The model under review builds one solid part; all positions refer to its coordinate system, in mm. A direction names the side the tool comes from. Round coordinates to 2 decimals unless told otherwise and drop trailing zeros. Write each loop counter-clockwise with the first axis right and the second up, starting at its lowest first coordinate (ties: lowest second). Pieces come first, ordered by that corner, then holes. Notation, with made-up numbers: (-18.5, 59) - (25.5, 59) arc R14 ccw to (25.5, 75) - close; hole circle Ø3 at (71.5, 46). An arc over 180 degrees is marked (long way). Return JSON: item names as keys, results as strings.
Autodesk Fusion 360 part; units mm, degrees
sketch "Sketch1" plane through (0, 0, 0) normal (0, 1, 0) x (1, 0, 0)
  line L0 (0, 0) -> (40.47, 0)
  line L1 (40.47, 0) -> (40.47, -39.36)
  line L2 (40.47, -39.36) -> (0, -39.36)
  line L3 (0, -39.36) -> (0, 0)
  line L4 (40.47, -9.96) -> (47.35, -9.96)
  line L5 (47.35, -9.96) -> (47.35, -12.36)
  line L6 (47.35, -12.36) -> (40.47, -12.36)
  line L7 (40.47, -29.96) -> (46.47, -29.96)
  line L8 (46.47, -29.96) -> (46.47, -33.96)
  line L9 (46.47, -33.96) -> (40.47, -33.96)
  line L10 (20.235, 0) -> (20.235, -39.36) construction
  line L11 (0, -9.96) -> (-6.88, -9.96)
  line L12 (-6.88, -9.96) -> (-6.88, -12.36)
  line L13 (-6.88, -12.36) -> (0, -12.36)
  dimension "d1" = 40.47
  dimension "d2" = 39.36
  dimension "d3" = 6.88
  dimension "d4" = 2.4
  dimension "d5" = 27
  dimension "d6" = 6
  dimension "d7" = 4
  dimension "d8" = 5.4
extrude "Extrude1" add sketch "Sketch1" along normal blind 19.6
sketch "Sketch2" plane through (0, 0, 0) normal (0, 0, -1) x (-1, 0, 0)
  line L0 (-40.47, 0) -> (0, 0)
  line L1 (0, 0) -> (0, 19.6)
  line L2 (0, 19.6) -> (-40.47, 19.6)
  line L3 (-40.47, 19.6) -> (-40.47, 0)
  circle A0 centre (-30.8, 9.8) radius 2.92
  line L4 (0, 9.8) -> (-40.47, 9.8) construction
  dimension "d11" = 5.84
  dimension "d12" = 9.67
extrude "Extrude2" add sketch "Sketch2" along normal blind 3.81 contours A0
sketch "Sketch3" plane through (0, 0, 9.96) normal (0, 0, -1) x (-1, 0, 0)
  line L0 (-47.35, 0) -> (-40.47, 0)
  line L1 (-40.47, 0) -> (-40.47, 19.6)
  line L2 (-40.47, 19.6) -> (-47.35, 19.6)
  line L3 (-47.35, 19.6) -> (-47.35, 0)
  circle A0 centre (-44.425, 14.58) radius 1.915
  circle A1 centre (-44.425, 5.02) radius 1.915
  line L4 (-40.47, 9.8) -> (-47.35, 9.8) construction
  line L5 (-40.47, 0) -> (-40.47, 19.6)
  line L6 (0, 0) -> (0, 19.6)
  line L7 (0, 0) -> (-40.47, 0)
  line L8 (-40.47, 19.6) -> (0, 19.6)
  line L9 (-20.235, 19.6) -> (-20.235, 0) construction
  dimension "d15" = 3.83
  dimension "d16" = 3.83
  dimension "d17" = 9.56
  dimension "d19" = 2.925
extrude "Extrude3" cut sketch "Sketch3" against normal up to surface (2.4 mm away) contours A0 | A1
ref_plane "WorkPlane1" through (20.235, 9.8, 4.98) normal (-1, 0, 0) x (0, 0, 1)
mirror "Mirror1" about plane through (20.235, 9.8, 4.98) normal (-1, 0, 0) of "Extrude3"
(1) Wall thickness on line 1 (Z direction, x = 35.5, y = 3.5); line 2 (X direction, y = 3.75, z = 28); line 3 (X direction, y = 2.5, z = 33.5): over which ranges is each line inside the solid? List them lowest first.
Filled in:
{"line 1": "z = 0 to 39.36", "line 2": "x = 0 to 40.47", "line 3": "x = 0 to 46.47"}
(2) Add section A-A (y = 5.02). Write out the cut boundary in (x, z).
Filled in:
{"outline": "(-6.88, 9.96) - (-5.87, 9.96) - (-5.87, 12.36) - (-6.88, 12.36) - close; (-2.04, 9.96) - (0, 9.96) - (0, 0) - (40.47, 0) - (40.47, 9.96) - (42.51, 9.96) - (42.51, 12.36) - (40.47, 12.36) - (40.47, 29.96) - (46.47, 29.96) - (46.47, 33.96) - (40.47, 33.96) - (40.47, 39.36) - (0, 39.36) - (0, 12.36) - (-2.04, 12.36) - close; (46.34, 9.96) - (47.35, 9.96) - (47.35, 12.36) - (46.34, 12.36) - close"}
(3) Clearance check with flat-ended pins moving along their axes: pin 1 Ø6 at (y, z) = (13, 25) entering from -X; pin 2 Ø8 at (y, z) = (12, 5.5) entering from +X; pin 3 Ø3.5 at (x, y) = (-3, 10) entering from -Z; pin 4 Ø3 at (x, y) = (-3.955, 14.58) entering from -Z. State where each tip first meets the part, or that it passes through.
Filled in:
{"pin 1": "stops at x = 0", "pin 2": "stops at x = 40.47", "pin 3": "stops at z = 9.96", "pin 4": "passes through"}
(4) Add section C-C (y = 17.75). Write out the cut boundary in (x, z), plus the area to 3 significant figures.
Filled in:
{"outline": "(-6.88, 9.96) - (0, 9.96) - (0, 0) - (40.47, 0) - (40.47, 9.96) - (47.35, 9.96) - (47.35, 12.36) - (40.47, 12.36) - (40.47, 29.96) - (46.47, 29.96) - (46.47, 33.96) - (40.47, 33.96) - (40.47, 39.36) - (0, 39.36) - (0, 12.36) - (-6.88, 12.36) - close", "area": "1,650 mm2"}
(5) Mouldability with a two-part tool opening along Y and no side actions: class faces 5 (the flat face through (20, 19.6, 19)), 6 (the flat face through (20, 0, 19)), 7 (the flat face through (-3, 10, 12.36)), 8 (the cylindrical face through (42.6, 15.16, 11.14)) as released by +Y, released by -Y, zero draft, split by the parting line, or undercut.
Filled in:
{"face 5": "released by +Y", "face 6": "released by -Y", "face 7": "zero draft", "face 8": "undercut"}
(6) For faces 1 (the flat face through (40.47, 10, 21)), 2 (the flat face through (44, 10, 33.96)), 3 (the flat face through (40.47, 10, 5)), 4 (the flat face through (0, 10, 26)), list the 3-axis set-ups (+Z, -Z, +X, -X, +Y, -Y) from which the entire face can be reached by the end or side of a thin tool; tool diameter is ignored.
Filled in:
{"face 1": "+X, +Y, -Y", "face 2": "+Z, +X, +Y, -Y", "face 3": "-Z, +X, +Y, -Y", "face 4": "+Z, -X, +Y, -Y"}
(7) Add section B-B (x = 30.8). Write out the cut boundary in (y, z).
Filled in:
{"outline": "(0, 0) - (6.88, 0) - (6.88, -3.81) - (12.72, -3.81) - (12.72, 0) - (19.6, 0) - (19.6, 39.36) - (0, 39.36) - close"}
(8) Add section D-D (x = 43.5). Write out the cut boundary in (y, z).
Filled in:
{"outline": "(0, 9.96) - (3.34, 9.96) - (3.34, 12.36) - (0, 12.36) - close; (0, 29.96) - (19.6, 29.96) - (19.6, 33.96) - (0, 33.96) - close; (6.7, 9.96) - (12.9, 9.96) - (12.9, 12.36) - (6.7, 12.36) - close; (16.26, 9.96) - (19.6, 9.96) - (19.6, 12.36) - (16.26, 12.36) - close"}
